Study the drawing (mm; zero at the part's minimum x, y, z) and answer. Give positions to 0.01 mm unless a question says otherwise; leave off trailing zeros. Write each loop counter-clockwise with the first axis right and the second up, starting at its lowest first coordinate (ties: lowest second). Pieces come first, ordered by that corner, then holes. Notation, with made-up numbers: (71, 22.5) - (109, 22.5) arc R15 ccw to (109, 36.5) - close; hole circle Ø2 at (23.5, 63.5). An arc over 180 degrees is marked (long way). Write each question's results on one line, items separated by ' | '. Start each with the question number.
Q1. Find the intervals of material crossed by probe 1 along X at (y, z) = (52.3, 59.37); probe 2 along X at (y, z) = (47, 2.9), in increasing order.
Q2. Flat-ended cylindrical pins translate along their axes: pin 1 Ø4 at (x, y) = (19.5, 35) entering from +Z; pin 2 Ø16 at (x, z) = (14, 42) entering from -Y; pin 3 Ø5.5 at (x, z) = (47, 59.37) entering from +Y. Find the tip coordinate at first contact, or state that the pin passes through.
Q3. Section B-B (x = 7) is taken. Determine the outline of the cut face in (y, z).
Q4. Section D-D (x = 19) is taken. Determine the outline of the cut face in (y, z), plus the area to 3 significant figures.
Q5. For a pull along Y with two mould halves and no side action, classify the marked faces 1, 2 and 3 as pulls with the +Y half, pulls with the -Y half, needs draft (parallel to the pull), parting line crosses it, or undercut.
Q6. Section A-A (z = 59.37) is taken. Determine the outline of the cut face in (x, y).
Q7. Section C-C (y = 7) is taken. Determine the outline of the cut face in (x, z), plus the area to 3 significant figures.
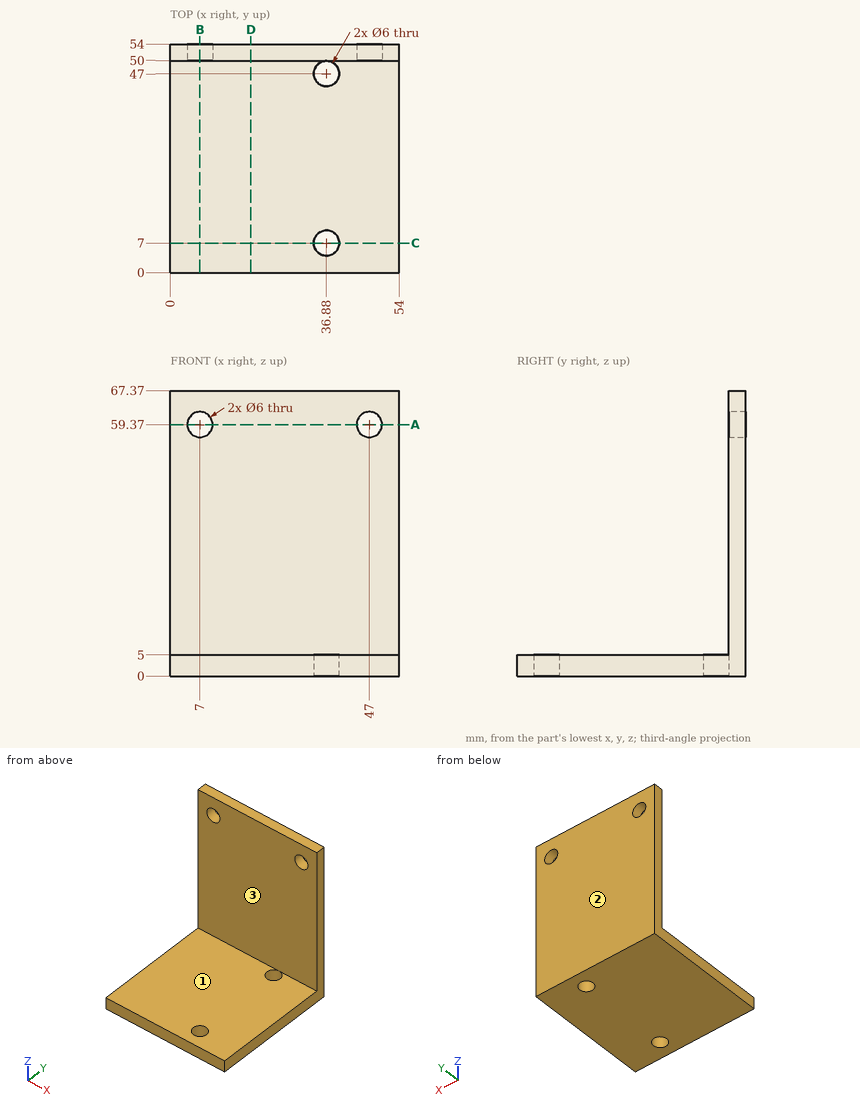
Answers below:
1) probe 1: x = 0 to 4, 10 to 44, 50 to 54 | probe 2: x = 0 to 33.88, 39.88 to 54
2) pin 1: stops at z = 5 | pin 2: stops at y = 50 | pin 3: passes through
3) outline: (0, 0) - (54, 0) - (54, 56.37) - (50, 56.37) - (50, 5) - (0, 5) - close; (50, 62.37) - (54, 62.37) - (54, 67.37) - (50, 67.37) - close
4) outline: (0, 0) - (54, 0) - (54, 67.37) - (50, 67.37) - (50, 5) - (0, 5) - close | area: 519 mm2
5) face 1: needs draft | face 2: pulls with the +Y half | face 3: pulls with the -Y half
6) outline: (0, 50) - (4, 50) - (4, 54) - (0, 54) - close; (10, 50) - (44, 50) - (44, 54) - (10, 54) - close; (50, 50) - (54, 50) - (54, 54) - (50, 54) - close
7) outline: (0, 0) - (33.88, 0) - (33.88, 5) - (0, 5) - close; (39.88, 0) - (54, 0) - (54, 5) - (39.88, 5) - close | area: 240 mm2
